```python
from build123d import *

# Parameters (mm, degrees)
SKETCH_1_W          = 260
SKETCH_1_H          = 100
EXTRUDE_1_DEPTH     = 3
FILLET_1_R          = 3
SKETCH_4_W          = 25
SKETCH_4_H          = 15
CUT_EXTRUDE_3_DEPTH = 500
FILLET_2_R          = 3
SKETCH_6_R          = 1.6
SKETCH_6_W          = 40
SKETCH_6_H          = 15
CUT_EXTRUDE_5_DEPTH = 10
FILLET_4_R          = 2
SKETCH_7_R          = 2.5
CUT_EXTRUDE_6_DEPTH = 10
SKETCH_8_R          = 2.6
CUT_EXTRUDE_7_DEPTH = 10
SKETCH_9_R          = 2.6
CUT_EXTRUDE_8_DEPTH = 10


with BuildPart() as part:
    # 草图1 → 凸台-拉伸1 (new body)
    with BuildSketch(Plane.XY):
        Rectangle(SKETCH_1_W, SKETCH_1_H)
    extrude(amount=EXTRUDE_1_DEPTH)

    # 圆角1
    fillet_1_edges = [part.edges().sort_by_distance(p)[0] for p in [
        (-130, 50, 1.5),
        (130, 50, 1.5),
        (130, -50, 1.5),
        (-130, -50, 1.5),
    ]]
    fillet(fillet_1_edges, radius=FILLET_1_R)

    # 草图4 → 切除-拉伸3 (cut)
    with BuildSketch(Plane.XY.offset(3)):
        with Locations((-82.5, -24.5)):
            Rectangle(SKETCH_4_W, SKETCH_4_H)
        with Locations((82.5, -24.5)):
            Rectangle(SKETCH_4_W, SKETCH_4_H)
    extrude(amount=-CUT_EXTRUDE_3_DEPTH, mode=Mode.SUBTRACT)

    # 圆角2
    fillet_2_edges = [part.edges().sort_by_distance(p)[0] for p in [
        (-95, -32, 1.5),
        (-95, -17, 1.5),
        (-70, -17, 1.5),
        (-70, -32, 1.5),
        (70, -17, 1.5),
        (95, -17, 1.5),
        (95, -32, 1.5),
        (70, -32, 1.5),
    ]]
    fillet(fillet_2_edges, radius=FILLET_2_R)

    # 草图6 → 切除-拉伸5 (cut)
    with BuildSketch(Plane.XY.offset(3)):
        with Locations((-65, 15)):
            Circle(SKETCH_6_R)
        with Locations((10, 15)):
            Circle(SKETCH_6_R)
        with Locations((10, -10)):
            Circle(SKETCH_6_R)
        with Locations((-65, -10)):
            Circle(SKETCH_6_R)
        with Locations((-17, 16.5)):
            Rectangle(SKETCH_6_W, SKETCH_6_H)
    extrude(amount=-CUT_EXTRUDE_5_DEPTH, mode=Mode.SUBTRACT)

    # 圆角4
    fillet_4_edges = [part.edges().sort_by_distance(p)[0] for p in [
        (-37, 9, 1.5),
        (-37, 24, 1.5),
        (3, 24, 1.5),
        (3, 9, 1.5),
    ]]
    fillet(fillet_4_edges, radius=FILLET_4_R)

    # 草图7 → 切除-拉伸6 (cut)
    with BuildSketch(Plane.XY.offset(3)):
        with Locations((46.5, 31.7)):
            Circle(SKETCH_7_R)
        with Locations((46.5, -10.3)):
            Circle(SKETCH_7_R)
    extrude(amount=-CUT_EXTRUDE_6_DEPTH, mode=Mode.SUBTRACT)

    # 草图8 → 切除-拉伸7 (cut)
    with BuildSketch(Plane.XY.offset(3)):
        with Locations((-108, 40)):
            Circle(SKETCH_8_R)
        with Locations((108, 40)):
            Circle(SKETCH_8_R)
        with Locations((-108, 22)):
            Circle(SKETCH_8_R)
        with Locations((108, 22)):
            Circle(SKETCH_8_R)
        with Locations((-95, 3.7)):
            Circle(SKETCH_8_R)
        with Locations((95, 3.7)):
            Circle(SKETCH_8_R)
    extrude(amount=-CUT_EXTRUDE_7_DEPTH, mode=Mode.SUBTRACT)

    # 草图9 → 切除-拉伸8 (cut)
    with BuildSketch(Plane.XY.offset(3)):
        with Locations((65, 3.7)):
            Circle(SKETCH_9_R)
    extrude(amount=-CUT_EXTRUDE_8_DEPTH, mode=Mode.SUBTRACT)


solid = part.part
```
Model file for the job. Use its own axes, mm. Coordinates: 2 decimals unless noted, no trailing zeros. Order: outer loops, then holes, each group sorted by start corner. A loop starts at its lowest first (then second) coordinate and runs counter-clockwise, first axis right, second up. Notation, with made-up numbers: (-28, 72) - (26, 72) arc R27 ccw to (26, 110) - close; hole circle Ø11 at (13, 65). An arc over 180 degrees is marked (long way). Return JSON: item names as keys, results as strings. Group by question number.
1) Saw through at B-B, the plane x = -10. Write the cut outline in (y, z).
2) Saw through at A-A, the plane y = 40. Write the cut outline in (x, z), plus the area to 3 significant figures.
3) Saw through at C-C, the plane x = 108. Write the cut outline in (y, z).
4) Saw through at D-D, the plane y = 3.7. Write the cut outline in (x, z).
5) Probe line 1 (Y direction, x = -108.5, z = 1.2); line 2 (Y direction, x = 10, z = 2.2); line 3 (Y direction, x = -9, z = 0.4). List the from-to ranges inside material, lowest first. Write a range as from..to.
6) Mould opens along X. For faces 1 (the cylindrical face through (62.4, 3.8, 1.5)), 2 (the flat face through (-2, 1, 0)), 3 (the cylindrical face through (-105.52, 22.78, 1.52)) say: released by +X, released by -X, zero draft, split by the parting line, or undercut.
Values found:
{
 "1": {"outline": "(-50, 0) - (9, 0) - (9, 3) - (-50, 3) - close; (24, 0) - (50, 0) - (50, 3) - (24, 3) - close"},
 "2": {"outline": "(-130, 0) - (-110.6, 0) - (-110.6, 3) - (-130, 3) - close; (-105.4, 0) - (105.4, 0) - (105.4, 3) - (-105.4, 3) - close; (110.6, 0) - (130, 0) - (130, 3) - (110.6, 3) - close", "area": "749 mm²"},
 "3": {"outline": "(-50, 0) - (19.4, 0) - (19.4, 3) - (-50, 3) - close; (24.6, 0) - (37.4, 0) - (37.4, 3) - (24.6, 3) - close; (42.6, 0) - (50, 0) - (50, 3) - (42.6, 3) - close"},
 "4": {"outline": "(-130, 0) - (-97.6, 0) - (-97.6, 3) - (-130, 3) - close; (-92.4, 0) - (62.4, 0) - (62.4, 3) - (-92.4, 3) - close; (67.6, 0) - (92.4, 0) - (92.4, 3) - (67.6, 3) - close; (97.6, 0) - (130, 0) - (130, 3) - (97.6, 3) - close"},
 "5": {"line 1": "y = -50..19.45, 24.55..37.45, 42.55..50", "line 2": "y = -50..-11.6, -8.4..13.4, 16.6..50", "line 3": "y = -50..9, 24..50"},
 "6": {"face 1": "undercut", "face 2": "zero draft", "face 3": "undercut"}
}
